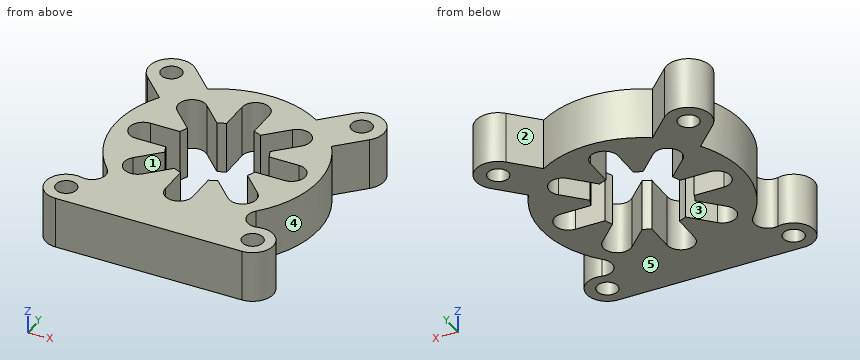
from build123d import *

# Parameters (mm, degrees)
CROQUIS1_R              = 6
SALIENTE_EXTRUIR2_DEPTH = 30


with BuildPart() as part:
    # Croquis1 → Saliente-Extruir2 (new body)
    # profile 1 of 2: a face of its own
    with BuildSketch(Plane.XY):
        with BuildLine():
            Line((45.961940777, 64.346717088), (31.501591743, 49.886368054))
            ThreePointArc((31.501591743, 49.886368054), (0, 59), (-31.501591743, 49.886368054))
            Line((-31.501591743, 49.886368054), (-45.961940777, 64.346717088))
            ThreePointArc((-45.961940777, 64.346717088), (-64.346717088, 64.346717088), (-64.346717088, 45.961940777))
            Line((-64.346717088, 45.961940777), (-49.886368054, 31.501591743))
            ThreePointArc((-49.886368054, 31.501591743), (0, -59), (49.886368054, 31.501591743))
            Line((49.886368054, 31.501591743), (64.346717088, 45.961940777))
            ThreePointArc((64.346717088, 45.961940777), (64.346717088, 64.346717088), (45.961940777, 64.346717088))
        make_face()
        with Locations((55.154328933, 55.154328933)):
            Circle(CROQUIS1_R, mode=Mode.SUBTRACT)
        with Locations((-55.154328933, 55.154328933)):
            Circle(CROQUIS1_R, mode=Mode.SUBTRACT)
        with BuildLine():
            ThreePointArc((12.577728279, 23.891436778), (10.332452674, 24.944747378), (8, 25.787593916))
            Line((8, 25.787593916), (8, 43))
            ThreePointArc((8, 43), (0, 51), (-8, 43))
            Line((-8, 43), (-8, 25.787593916))
            ThreePointArc((-8, 25.787593916), (-10.332452674, 24.944747378), (-12.577728279, 23.891436778))
            Line((-12.577728279, 23.891436778), (-24.748737342, 36.062445841))
            ThreePointArc((-24.748737342, 36.062445841), (-36.062445841, 36.062445841), (-36.062445841, 24.748737342))
            Line((-36.062445841, 24.748737342), (-23.891436778, 12.577728279))
            ThreePointArc((-23.891436778, 12.577728279), (-24.944747378, 10.332452674), (-25.787593916, 8))
            Line((-25.787593916, 8), (-43, 8))
            ThreePointArc((-43, 8), (-51, 0), (-43, -8))
            Line((-43, -8), (-25.787593916, -8))
            ThreePointArc((-25.787593916, -8), (-24.944747378, -10.332452674), (-23.891436778, -12.577728279))
            Line((-23.891436778, -12.577728279), (-36.062445841, -24.748737342))
            ThreePointArc((-36.062445841, -24.748737342), (-36.062445841, -36.062445841), (-24.748737342, -36.062445841))
            Line((-24.748737342, -36.062445841), (-12.577728279, -23.891436778))
            ThreePointArc((-12.577728279, -23.891436778), (-10.332452674, -24.944747378), (-8, -25.787593916))
            Line((-8, -25.787593916), (-8, -43))
            ThreePointArc((-8, -43), (0, -51), (8, -43))
            Line((8, -43), (8, -25.787593916))
            ThreePointArc((8, -25.787593916), (10.332452674, -24.944747378), (12.577728279, -23.891436778))
            Line((12.577728279, -23.891436778), (24.748737342, -36.062445841))
            ThreePointArc((24.748737342, -36.062445841), (36.062445841, -36.062445841), (36.062445841, -24.748737342))
            Line((36.062445841, -24.748737342), (23.891436778, -12.577728279))
            ThreePointArc((23.891436778, -12.577728279), (24.944747378, -10.332452674), (25.787593916, -8))
            Line((25.787593916, -8), (43, -8))
            ThreePointArc((43, -8), (51, 0), (43, 8))
            Line((43, 8), (25.787593916, 8))
            ThreePointArc((25.787593916, 8), (24.944747378, 10.332452674), (23.891436778, 12.577728279))
            Line((23.891436778, 12.577728279), (36.062445841, 24.748737342))
            ThreePointArc((36.062445841, 24.748737342), (36.062445841, 36.062445841), (24.748737342, 36.062445841))
            Line((24.748737342, 36.062445841), (12.577728279, 23.891436778))
        make_face(mode=Mode.SUBTRACT)
    # profile 2 of 2: a face of its own
    with BuildSketch(Plane.XY):
        with BuildLine():
            ThreePointArc((43.213377787, -40.16968982), (0, -59), (-43.213377787, -40.16968982))
            ThreePointArc((-43.213377787, -40.16968982), (-42.192314412, -49.697929449), (-51.043691305, -53.369856454))
            ThreePointArc((-51.043691305, -53.369856454), (-65.907176881, -63.510322611), (-54, -77))
            Line((-54, -77), (-0.009258466, -77))
            Line((-0.009258466, -77), (0.009258466, -77))
            Line((0.009258466, -77), (54, -77))
            ThreePointArc((54, -77), (65.907176881, -63.510322611), (51.043691305, -53.369856454))
            ThreePointArc((51.043691305, -53.369856454), (42.192314412, -49.697929449), (43.213377787, -40.16968982))
        make_face()
        with Locations((-54, -65)):
            Circle(CROQUIS1_R, mode=Mode.SUBTRACT)
        with Locations((54, -65)):
            Circle(CROQUIS1_R, mode=Mode.SUBTRACT)
    extrude(amount=SALIENTE_EXTRUIR2_DEPTH)


solid = part.part
The model under review builds one solid part; all positions refer to its coordinate system, in mm. Face numbers are marked on the shaded views. A direction names the side the tool comes from. Give positions to 0.01 mm unless a question says otherwise; leave off trailing zeros. Order: outer loops, then holes, each group sorted by start corner. A loop starts at its lowest first (then second) coordinate and runs counter-clockwise, first axis right, second up. Notation, with made-up numbers: M -34.5,-1.75 L 13.5,-1.75 A24 cw 13.5,19.25 Z; hole C 62.5,10 d6. An arc over 180 degrees is marked long. One line per question, with ' | ' between items. Start each with the question number.
1) Consider section A-A, the plane y = 0. Give the boundary of the cut face in (x, z), then the cut area to 3 significant figures.
2) Clearance check with flat-ended pins moving along their axes: P1, Ø4, axis at x = -1, z = 27, coming from the +Y side; P2, Ø8, axis at y = -18.5, z = 14, coming from the +X side; P3, Ø5, axis at y = 36.5, z = 16.5, coming from the -X side; P4, Ø7, axis at x = -55.15, y = 55.15, coming from the +Z side. State where each tip first meets the part, or that it passes through.
3) Consider section C-C, the plane y = -65. Give the boundary of the cut face in (x, z), then the cut area to 3 significant figures.
4) Consider section D-D, the plane y = -31. Give the boundary of the cut face in (x, z).
5) Mouldability with a two-part tool opening along X and no side actions: class the marked faces 3, 4 and 5 as pulls with the +X half, pulls with the -X half, needs draft (parallel to the pull), parting line crosses it, or undercut.
6) Wall thickness on L1, parallel to Y at x = -36, z = 19; L2, parallel to Y at x = -36.5, z = 19; L3, parallel to Y at x = 54, z = 13.75: over which ranges is each line inside the solid? List them lowest first. Write a range as from..to.
7) For the marked faces 1 and 2, list the 3-axis set-ups (+Z, -Z, +X, -X, +Y, -Y) from which the entire face can be reached by the end or side of a thin tool; tool diameter is ignored.
8) Consider section B-B, the plane x = -2. Give the boundary of the cut face in (y, z).
Found:
1) outline: M -59,0 L -51,0 L -51,30 L -59,30 Z; M 51,0 L 59,0 L 59,30 L 51,30 Z | area: 480 mm²
2) P1: stops at y = 59 | P2: stops at x = 57.19 | P3: stops at x = -57.38 | P4: passes through
3) outline: M -66,0 L -60,0 L -60,30 L -66,30 Z; M -48,0 L 48,0 L 48,30 L -48,30 Z; M 60,0 L 66,0 L 66,30 L 60,30 Z | area: 3,240 mm²
4) outline: M -50.2,0 L -38.38,0 L -38.38,30 L -50.2,30 Z; M -19.69,0 L -8,0 L -8,30 L -19.69,30 Z; M 8,0 L 19.69,0 L 19.69,30 L 8,30 Z; M 38.38,0 L 50.2,0 L 50.2,30 L 38.38,30 Z
5) face 3: undercut | face 4: pulls with the +X half | face 5: needs draft
6) L1: y = -77..-36.12, -24.69..-8, 8..24.69, 36.12..54.38 | L2: y = -77..-35.59, -25.22..-8, 8..25.22, 35.59..54.88 | L3: y = -77..-71, -59..-53, -23.77..23.77, 35.62..49.27, 61.04..68.1
7) face 1: +Z, -Z | face 2: +Z, -Z, +Y
8) outline: M -77,0 L -50.75,0 L -50.75,30 L -77,30 Z; M 50.75,0 L 58.97,0 L 58.97,30 L 50.75,30 Z
